Autodesk Inventor part; units mm, degrees
ref_plane "YZ Plane" through (0, 0, 0) normal (1, 0, 0) x (0, 1, 0)
ref_plane "XZ Plane" through (0, 0, 0) normal (0, 1, 0) x (-1, 0, 0)
ref_plane "XY Plane" through (0, 0, 0) normal (0, 0, 1) x (1, 0, 0)
sketch "Sketch1" plane through (0, 0, 0) normal (0, 1, 0) x (-1, 0, 0)
  line L0 (0, 0) -> (57.15, 0)
  line L1 (57.15, 0) -> (57.15, -19.05)
  line L2 (57.15, -19.05) -> (19.05, -19.05)
  line L3 (19.05, -19.05) -> (19.05, -59.69)
  line L4 (19.05, -59.69) -> (0, -59.69)
  line L5 (0, -59.69) -> (0, 0)
  circle A0 centre (28.575, -9.525) radius 2.5527
  circle A1 centre (47.625, -9.525) radius 2.5527
  line L6 (19.05, -19.05) -> (0, 0) construction
  circle A2 centre (9.525, -28.575) radius 2.5527
  circle A3 centre (9.525, -47.625) radius 2.5527
  circle A4 centre (9.525, -9.525) radius 2.413
  point P0 (57.15, -9.525)
  dimension "d0" = 19.05
  dimension "d1" = 19.05
  dimension "d2" = 59.69
  dimension "d3" = 57.15
  dimension "d4" = 5.1054
  dimension "d5" = 28.575
  dimension "d6" = 19.05
  dimension "d19" = 4.826
extrude "Extrusion1" add sketch "Sketch1" along normal mid plane 19.05
thread "Thread1"
thread "Thread2"
thread "Thread3"
thread "Thread4"
thread "Thread5"
properties part number "STRU_004_DoubleBillet_90_2.25in" material "Aluminum 6061"
Verification items for the finished model (mm, model axes). A direction names the side the tool comes from. Give positions to 0.01 mm unless a question says otherwise; leave off trailing zeros. Order: outer loops, then holes, each group sorted by start corner. A loop starts at its lowest first (then second) coordinate and runs counter-clockwise, first axis right, second up. Notation, with made-up numbers: M -34.5,55.25 L 14.5,55.25 A18 ccw 14.5,61.25 Z; hole C 74,-10.75 d9. An arc over 180 degrees is marked long. Use one line per item in the form item = value. Start each with the question number.
Q1. Section check A-A (x = -46). Enter the section's corners in (y, z) (3 decimals).
Q2. Section check B-B (x = -10.5). Enter the section's corners in (y, z) (3 decimals).
Q3. Access from +Z, -Z, +X, -X, +Y, -Y to the whole of each face (thin tool, end or side, straight path). Record for faces 1 (the flat face through (-15, -9.525, -23)), 2 (the flat face through (-38, 0, -19.05)).
Q4. Go/stop test with flat-tipped pins: pin 1 Ø3 at (y, z) = (-4, -52) entering from -X; pin 2 Ø4.5 at (x, z) = (-47.625, -9.525) entering from -Y; pin 3 Ø5.5 at (x, y) = (-41.5, 0) entering from -Z. Record where each tip stops, or that it passes through.
Q5. Section check D-D (z = -52.5). Enter the section's corners in (x, y) (3 decimals), then the cut area to 3 significant figures.
Q6. Mould release check, pull along X, two halves, no side actions. Record for faces 3 (the cylindrical face through (-28.022, -0.133, -7.033)), 4 (the flat face through (-57.15, 0, -9)), 5 (the flat face through (-10, 0, -59.69)): +X half, -X half, draft (parallel to the pull), parting line (faces both ways), or undercut.
Q7. Section check C-C (y = 3.5). Enter the section's corners in (x, z) (3 decimals), then the cut area to 3 significant figures.
Q8. Scan lines: line 1 along X through (y, z) = (-3.75, -9.5); line 2 along X through (y, z) = (-1, -21); line 3 along Z through (x, y) = (-49, -2.5). Record each from-to range of solid material in increasing order. Write a range as [from, to].
Evaluation:
q1.outline = M -9.525,-19.05 L 9.525,-19.05 L 9.525,-11.494 L -9.525,-11.494 Z; M -9.525,-7.556 L 9.525,-7.556 L 9.525,0 L -9.525,0 Z
q2.outline = M -9.525,-59.69 L 9.525,-59.69 L 9.525,-49.984 L -9.525,-49.984 Z; M -9.525,-45.266 L 9.525,-45.266 L 9.525,-30.934 L -9.525,-30.934 Z; M -9.525,-26.216 L 9.525,-26.216 L 9.525,-11.732 L -9.525,-11.732 Z; M -9.525,-7.318 L 9.525,-7.318 L 9.525,0 L -9.525,0 Z
q3.face_1 = +Z, -Z, +X, -X, -Y
q3.face_2 = -Z, -X, +Y, -Y
q4.pin_1 = -19.05
q4.pin_2 = through
q4.pin_3 = -19.05
q5.outline = M -19.05,-9.525 L 0,-9.525 L 0,9.525 L -19.05,9.525 Z
q5.area = 363 mm2
q6.face_3 = undercut
q6.face_4 = -X half
q6.face_5 = draft
q7.outline = M -57.15,-19.05 L -19.05,-19.05 L -19.05,-59.69 L 0,-59.69 L 0,0 L -57.15,0 Z; hole C -47.625,-9.525 d5.105; hole C -28.575,-9.525 d5.105; hole C -9.525,-47.625 d5.105; hole C -9.525,-28.575 d5.105; hole C -9.525,-9.525 d4.826
q7.area = 1,760 mm2
q8.line_1 = [-57.15, -50.18], [-45.07, -31.13], [-26.02, -11.94], [-7.11, 0]
q8.line_2 = [-19.05, 0]
q8.line_3 = [-19.05, -11.68], [-7.37, 0]
